Could you check a few things on this model? Use its own coordinates, in mm. Face numbers are marked on the shaded views. A direction names the side the tool comes from. Coordinates: 2 decimals unless noted, no trailing zeros. Loops run counter-clockwise (first coordinate to the right, second up) from the corner with the lowest first, then second, coordinate; pieces in that order, holes last. Notation, with made-up numbers: (66.25, 85.5) - (97.25, 85.5) arc R38 ccw to (97.25, 123.5) - close; hole circle Ø8 at (3.5, 19). An arc over 180 degrees is marked (long way). One line per question, with ' | ' between items. Start each with the question number.
1. Please list where these lines run through material, in increasing order: L1, parallel to Z at x = -9, y = 350; L2, parallel to Z at x = -0.5, y = 51.5; L3, parallel to X at y = 237, z = -90. Write a range as [from, to].
2. I want a section at A-A, the plane y = 370.5. Write out the boundary of the cut face in (x, z).
3. I want a section at D-D, the plane x = -8. Write out the boundary of the cut face in (y, z), then the cut area to 3 significant figures.
4. I want a section at C-C, the plane z = -72. Write out the boundary of the cut face in (x, y).
5. We'd pull the mould along Z, two halves only. Please class the marked faces 5, 6, 7 and 8: pulls with the +Z half, pulls with the -Z half, needs draft (parallel to the pull), parting line crosses it, or undercut.
6. I want a section at B-B, the plane x = 48.5. Write out the boundary of the cut face in (y, z), then the cut area to 3 significant figures.
7. I'm going to push flat-ended pins straight in: P1, Ø2, axis at y = 106, z = 21.5, coming from the +X side; P2, Ø1.5, axis at x = -23.5, y = 125, coming from the -Z side; P3, Ø8, axis at x = 17.5, z = 52, coming from the +Y side. Where does each tip first touch, or does it pass through?
8. Which directions (+Z, -Z, +X, -X, +Y, -Y) give clear straight access to the entire face, cutting with the end or side of a thin tool? Please do the marked faces 1, 2, 3 and 4.
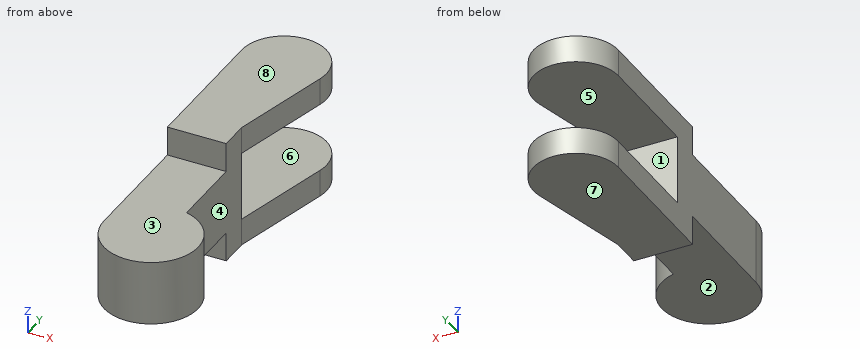
from build123d import *

# Parameters (mm, degrees)
BOSS_EXTRUDE1_DEPTH     = 105
CUT_EXTRUDE1_DEPTH      = 539.431982705
CUT_EXTRUDE1_DEPTH_BACK = 539.431982705
SKETCH2_W               = 118
SKETCH2_H               = 265
SKETCH2_W_2             = 50
SKETCH2_H_2             = 287


with BuildPart() as part:
    # Sketch1 → Boss-Extrude1 (new, symmetric)
    with BuildSketch(Plane.XY):
        with BuildLine():
            Line((-80, 0), (-80, 450))
            ThreePointArc((-80, 450), (0.428269124, 521.504994788), (62.026785544, 433.259351673))
            Line((62.026785544, 433.259351673), (20, 257.459666924))
            Line((20, 257.459666924), (20, 77.459666924))
            ThreePointArc((20, 77.459666924), (48.989794856, -63.245553203), (-80, 0))
        make_face()
    extrude(amount=BOSS_EXTRUDE1_DEPTH, both=True)

    # Sketch2 → Cut-Extrude1 (cut, two sides: drawn at the far end of the back side and taken through both)
    with BuildSketch(Plane(origin=(0, 0, 0), x_dir=(0, 0, -1), z_dir=(1, 0, 0)).offset(-CUT_EXTRUDE1_DEPTH_BACK)):
        with Locations((0, 389.5)):
            Rectangle(SKETCH2_W, SKETCH2_H)
        with Locations((-80, 63.5)):
            Rectangle(SKETCH2_W_2, SKETCH2_H_2)
        with Locations((80, 63.5)):
            Rectangle(SKETCH2_W_2, SKETCH2_H_2)
    extrude(amount=CUT_EXTRUDE1_DEPTH + CUT_EXTRUDE1_DEPTH_BACK, mode=Mode.SUBTRACT)


solid = part.part
Results are:
1) L1: z = [-105, -59], [59, 105] | L2: z = [-55, 55] | L3: x = [-80, 20]
2) outline: (-80, -105) - (47.02, -105) - (47.02, -59) - (-80, -59) - close; (-80, 59) - (47.02, 59) - (47.02, 105) - (-80, 105) - close
3) outline: (-79.6, -55) - (207, -55) - (207, -105) - (522, -105) - (522, -59) - (257, -59) - (257, 59) - (522, 59) - (522, 105) - (207, 105) - (207, 55) - (-79.6, 55) - close | area: 66,400 mm2
4) outline: (-80, 207) - (20, 207) - (20, 257.46) - (62.03, 433.26) arc R72 ccw (long way) to (-80, 450) - close
5) face 5: undercut | face 6: undercut | face 7: pulls with the -Z half | face 8: pulls with the +Z half
6) outline: (-63.62, -55) - (63.62, -55) - (63.62, 55) - (-63.62, 55) - close; (376.68, -105) - (494.63, -105) - (494.63, -59) - (376.68, -59) - close; (376.68, 59) - (494.63, 59) - (494.63, 105) - (376.68, 105) - close | area: 24,800 mm2
7) P1: stops at x = 20 | P2: stops at z = -55 | P3: stops at y = 257
8) face 1: +X, -X, +Y | face 2: -Z, +X, -X, -Y | face 3: +Z, +X, -X, -Y | face 4: +Z, -Z, +X
